Read the model definition and answer for the solid it produces. Units are mm, in the model's axes. A direction names the side the tool comes from. Coordinates: 2 decimals unless noted, no trailing zeros. Order: outer loops, then holes, each group sorted by start corner. A loop starts at its lowest first (then second) coordinate and runs counter-clockwise, first axis right, second up. Notation, with made-up numbers: (-13, 11) - (23, 11) arc R20 cw to (23, 21) - close; hole circle Ø11 at (-3, 71). An arc over 180 degrees is marked (long way). Use one line per item in the form item = value.
```python
from build123d import *

# Parameters (mm, degrees)
BOSS_EXTRUDE1_DEPTH      = 311.5
BOSS_EXTRUDE1_DEPTH_BACK = 61.5
SKETCH2_R                = 4.34
SKETCH2_W                = 30
SKETCH2_H                = 24
SKETCH2_H_2              = 6
CORTAR_EXTRUIR1_DEPTH    = 30
CORTAR_EXTRUIR3_REACH    = 65
REDONDEO1_R              = 5


with BuildPart() as part:
    # Sketch1 → Boss-Extrude1 (new body, two sides)
    with BuildSketch(Plane(origin=(0, 0, 0), x_dir=(0, 0, -1), z_dir=(1, 0, 0))) as boss_extrude1_sk:
        Polygon((0, 0), (6, 0), (6, 57), (119, 57), (119, 0), (125, 0), (125, 63), (0, 63), align=None)
    extrude(amount=BOSS_EXTRUDE1_DEPTH)
    extrude(boss_extrude1_sk.sketch, amount=-BOSS_EXTRUDE1_DEPTH_BACK)

    # Sketch2 → Cortar-Extruir1 (cut)
    with BuildSketch(Plane(origin=(0, 0, -125), x_dir=(-1, 0, 0), z_dir=(0, 0, -1))):
        Polygon((-311.5, 0), (-266.5, 0), (-266.5, 16), (-283.5, 16), (-283.5, 6.4), (-311.5, 6.4), align=None)
        with Locations((-277.52, 10.9)):
            Circle(SKETCH2_R, mode=Mode.SUBTRACT)
        with Locations((-277.52, 10.9)):
            Circle(SKETCH2_R)
        with Locations((-125, 45)):
            Rectangle(SKETCH2_W, SKETCH2_H)
        with Locations((-125, 60)):
            Rectangle(SKETCH2_W, SKETCH2_H_2)
        Polygon((16.5, 16), (16.5, 0), (61.5, 0), (61.5, 6.4), (33.5, 6.4), (33.5, 16), align=None)
    extrude(amount=-CORTAR_EXTRUIR1_DEPTH, mode=Mode.SUBTRACT)

    # Croquis1 → Cortar-Extruir3 (cut, up to next)
    with BuildSketch(Plane(origin=(0, 63, 0), x_dir=(1, 0, 0), z_dir=(0, 1, 0)), mode=Mode.PRIVATE) as cortar_extruir3_sk1:
        Polygon((-31.5, 95), (-31.5, 30), (281.5, 30), (281.5, 95), (170, 95), (140, 95), (110, 95), (80, 95), align=None)
    cortar_extruir3_tool1 = extrude(cortar_extruir3_sk1.sketch, amount=-CORTAR_EXTRUIR3_REACH, mode=Mode.PRIVATE) & part.part
    add(cortar_extruir3_tool1.solids().sort_by_distance((125, 63, -62.5))[0], mode=Mode.SUBTRACT)

    # Redondeo1
    redondeo1_edges = [part.edges().sort_by_distance(p)[0] for p in [
        (-16.5, 16, -122),
        (-33.5, 16, -122),
        (-31.5, 60, -95),
        (281.5, 60, -95),
        (281.5, 60, -30),
        (-31.5, 60, -30),
        (283.5, 16, -122),
        (266.5, 16, -122),
    ]]
    fillet(redondeo1_edges, radius=REDONDEO1_R)


solid = part.part
```
(1) Which of the six approach directions +Z, -Z, +X, -X, +Y, -Y give full straight-line access (tool end or side, diameter ignored) to faces 1 (the flat face through (-48, 6.4, -122)), 2 (the flat face through (110, 54, -120)), 3 (the flat face through (-25, 16, -122)), 4 (the flat face through (123, 60, -30)), 5 (the flat face through (128, 57, -24))?
Answer list:
face_1 = -Z, -X, -Y
face_2 = -Z, +Y
face_3 = -Z, -Y
face_4 = +Y, -Y
face_5 = +X, -X, -Y
(2) Section C-C, the plane z = -62 is taken. Write down the section's boundary in (x, y), then the cut area to 3 significant figures.
Answer list:
outline = (-61.5, 57) - (-31.5, 57) - (-31.5, 63) - (-61.5, 63) - close; (281.5, 57) - (311.5, 57) - (311.5, 63) - (281.5, 63) - close
area = 360 mm2
(3) Section B-B, the plane x = 230.5 is taken. Write down the section's boundary in (y, z), then the cut area to 3 significant figures.
Answer list:
outline = (0, -125) - (63, -125) - (63, -95) - (57, -95) - (57, -119) - (0, -119) - close; (0, -6) - (57, -6) - (57, -30) - (63, -30) - (63, 0) - (0, 0) - close
area = 1,040 mm2
(4) Straight lines are drawn through the part: L1, parallel to Z at x = 61, y = 35.5; L2, parallel to Y at x = -2, z = -107. For each, find the intervals that lie inside material, in ascending order.
Answer list:
L1 = -125 to -119, -6 to 0
L2 = 57 to 63
(5) Section A-A, the plane y = 43 is taken. Write down the section's boundary in (x, z).
Answer list:
outline = (-61.5, -125) - (110, -125) - (110, -119) - (-61.5, -119) - close; (-61.5, -6) - (311.5, -6) - (311.5, 0) - (-61.5, 0) - close; (140, -125) - (311.5, -125) - (311.5, -119) - (140, -119) - close
(6) The mould has two halves that part along X. Classify faces 6 (the flat face through (128, 0, -3)), 7 (the flat face through (-61.5, 57.3, -62.2)), 8 (the flat face through (281.5, 60, -62)): +X half, -X half, draft (parallel to the pull), parting line (faces both ways), or undercut.
Answer list:
face_6 = draft
face_7 = -X half
face_8 = undercut
(7) Section D-D, the plane z = -15.5 is taken. Write down the section's boundary in (x, y).
Answer list:
outline = (-61.5, 57) - (311.5, 57) - (311.5, 63) - (-61.5, 63) - close
(8) Given pin 1 Ø6.5 at (x, z) = (-25.5, -122.5) entering from -Y; pin 2 Ø3 at (x, y) = (219.5, 60) entering from +Z; pin 3 Ø6.5 at (x, z) = (118.5, -122) entering from +Y; pin 4 Ø8 at (x, z) = (162.5, -95) entering from -Y, each flat-ended and moving along its own axis, determine where each tip first touches the part or whether it passes through.
Answer list:
pin_1 = 15.99
pin_2 = 0
pin_3 = 33
pin_4 = 57
